Design review of the part built by this model. Coordinates are the model's own, in mm. Face numbers are marked on the shaded views. A direction names the side the tool comes from. Coordinates: 2 decimals unless noted, no trailing zeros. Loops run counter-clockwise (first coordinate to the right, second up) from the corner with the lowest first, then second, coordinate; pieces in that order, holes last. Notation, with made-up numbers: M 0.25,73.25 L 41.25,73.25 A20 ccw 41.25,94.25 Z; hole C 56,-34.5 d8. An arc over 180 degrees is marked long. One line per item, written item: value.
```python
from build123d import *

# Parameters (mm, degrees)
SKETCH1_W           = 120
SKETCH1_H           = 80
BOSS_EXTRUDE1_DEPTH = 10
SKETCH2_R           = 17.5
SKETCH2_R_2         = 12.5
BOSS_EXTRUDE2_DEPTH = 18
FILLET1_R           = 20
FILLET2_R           = 5


with BuildPart() as part:
    # Sketch1 → Boss-Extrude1 (new body)
    with BuildSketch(Plane(origin=(0, 0, 0), x_dir=(1, 0, 0), z_dir=(0, 1, 0))):
        with Locations((60, 40)):
            Rectangle(SKETCH1_W, SKETCH1_H)
    extrude(amount=BOSS_EXTRUDE1_DEPTH)

    # Sketch2 → Boss-Extrude2 (add)
    # profile 1 of 4: a face of its own
    with BuildSketch(Plane(origin=(0, 10, 0), x_dir=(1, 0, 0), z_dir=(0, 1, 0))):
        with BuildLine():
            Line((49.270509831, 45), (70.729490169, 45))
            ThreePointArc((70.729490169, 45), (71.734561363, 47.596113781), (73.138593384, 50))
            Line((73.138593384, 50), (46.861406616, 50))
            ThreePointArc((46.861406616, 50), (48.265438637, 47.596113781), (49.270509831, 45))
        make_face()
    # profile 2 of 4: a face of its own
    with BuildSketch(Plane(origin=(0, 10, 0), x_dir=(1, 0, 0), z_dir=(0, 1, 0))):
        with Locations((32.5, 40)):
            Circle(SKETCH2_R)
        with Locations(Location((32.5, 40, 0), (0, 0, 270))):
            Circle(SKETCH2_R_2, mode=Mode.SUBTRACT)
    # profile 3 of 4: a face of its own
    with BuildSketch(Plane(origin=(0, 10, 0), x_dir=(1, 0, 0), z_dir=(0, 1, 0))):
        with BuildLine():
            ThreePointArc((73.138593384, 30), (71.734561363, 32.403886219), (70.729490169, 35))
            Line((70.729490169, 35), (49.270509831, 35))
            ThreePointArc((49.270509831, 35), (48.265438637, 32.403886219), (46.861406616, 30))
            Line((46.861406616, 30), (73.138593384, 30))
        make_face()
    # profile 4 of 4: a face of its own
    with BuildSketch(Plane(origin=(0, 10, 0), x_dir=(1, 0, 0), z_dir=(0, 1, 0))):
        with Locations((87.5, 40)):
            Circle(SKETCH2_R)
        with Locations(Location((87.5, 40, 0), (0, 0, 270))):
            Circle(SKETCH2_R_2, mode=Mode.SUBTRACT)
    extrude(amount=BOSS_EXTRUDE2_DEPTH)

    # Fillet1
    fillet1_edges = [part.edges().sort_by_distance(p)[0] for p in [
        (0, 5, -80),
        (120, 5, -80),
        (120, 5, 0),
        (0, 5, 0),
    ]]
    fillet(fillet1_edges, radius=FILLET1_R)

    # Fillet2
    fillet2_edges = [part.edges().sort_by_distance(p)[0] for p in [
        (0, 10, -40),
        (60, 10, -80),
        (60, 10, 0),
        (120, 10, -40),
        (5.857864376, 10, -5.857864376),
        (114.142135624, 10, -5.857864376),
        (114.142135624, 10, -74.142135624),
        (5.857864376, 10, -74.142135624),
    ]]
    fillet(fillet2_edges, radius=FILLET2_R)


solid = part.part
```
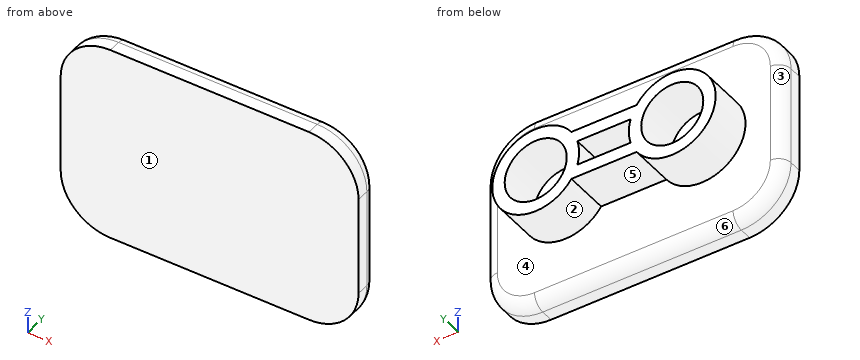
(1) Mouldability with a two-part tool opening along X and no side actions: class the marked faces 1, 2 and 3 as released by +X, released by -X, zero draft, split by the parting line, or undercut.
Reply:
face 1: zero draft
face 2: undercut
face 3: released by -X
(2) To check wall thickness, follow line 1 along Y through (x, z) = (26.5, -32); line 2 along X through (y, z) = (12, -56); line 3 along Z through (x, y) = (82, 22). State the ranges of each line that lie inside material, in increasing order. Write a range as [from, to].
Reply:
line 1: y = [0, 10]
line 2: x = [25.41, 39.59], [80.41, 94.59]
line 3: z = [-56.61, -51.22], [-28.78, -23.39]
(3) Insertion check: pin 1 (5.5 mm diameter, centred on x = 60, y = 21, fed in from +Z); pin 2 (3 mm diameter, centred on y = 24.5, z = -60, fed in from -X); pin 3 (2 mm diameter, centred on y = 15, z = -55.5, fed in from +X); pin 4 (1 mm diameter, centred on x = 49, z = -15, fed in from +Y). Each pin has a flat end and moves straight along its axis. Give the tip position at first contact, or say it passes through.
Reply:
pin 1: stops at z = -30
pin 2: passes through
pin 3: stops at x = 97.3
pin 4: stops at y = 10
(4) We need section B-B on x = 87.5. State the section outline as (y, z) points, then the cut area to 3 significant figures.
Reply:
outline: M 0,-80 L 5,-80 A5 ccw 10,-75 L 10,-57.5 L 28,-57.5 L 28,-52.5 L 10,-52.5 L 10,-27.5 L 28,-27.5 L 28,-22.5 L 10,-22.5 L 10,-5 A5 ccw 5,0 L 0,0 Z
area: 969 mm2
(5) We need section A-A on y = 25.5. State the section outline as (x, z) points, then the cut area to 3 significant figures.
Reply:
outline: M 46.86,-50 L 73.14,-50 A17.5 ccw long 73.14,-30 L 46.86,-30 A17.5 ccw long Z; hole C 32.5,-40 d25; hole M 49.27,-45 L 70.73,-45 A17.5 cw 70.73,-35 L 49.27,-35 A17.5 cw Z; hole C 87.5,-40 d25
area: 1,180 mm2
(6) We need section C-C on z = -40. State the section outline as (x, y) points.
Reply:
outline: M 0,0 L 120,0 L 120,5 A5 ccw 115,10 L 105,10 L 105,28 L 100,28 L 100,10 L 75,10 L 75,28 L 70,28 L 70,10 L 50,10 L 50,28 L 45,28 L 45,10 L 20,10 L 20,28 L 15,28 L 15,10 L 5,10 A5 ccw 0,5 Z
(7) We need section D-D on y = 7.5. State the section outline as (x, z) points.
Reply:
outline: M 0.67,-60 A19.33 ccw 20,-79.33 L 100,-79.33 A19.33 ccw 119.33,-60 L 119.33,-20 A19.33 ccw 100,-0.67 L 20,-0.67 A19.33 ccw 0.67,-20 Z
(8) Tool access review of the marked faces 4, 5 and 6: name each direction out of +Z, -Z, +X, -X, +Y, -Y from which nothing blocks a thin tool from reaching the whole face with its end or side.
Reply:
face 4: +Y
face 5: -Z, +Y
face 6: -Z, +X, -X, +Y
